from build123d import *

# Parameters (mm, degrees)
BOSS_EXTRUDE1_DEPTH = 3.175
SKETCH3_R           = 10.16
CUT_EXTRUDE1_DEPTH  = 281.570134948
LPATTERN1_COUNT     = 8
LPATTERN1_PITCH     = 35.56


with BuildPart() as part:
    # Sketch1 → Boss-Extrude1 (new body)
    with BuildSketch(Plane(origin=(0, 0, 0), x_dir=(1, 0, 0), z_dir=(0, 1, 0))):
        with BuildLine():
            Line((0, 25.4), (-254, 25.4))
            ThreePointArc((-254, 25.4), (-279.4, 0), (-254, -25.4))
            Line((-254, -25.4), (0, -25.4))
            ThreePointArc((0, -25.4), (25.4, 0), (0, 25.4))
        make_face()
    extrude(amount=BOSS_EXTRUDE1_DEPTH)

    # Sketch3 → Cut-Extrude1 (cut, through all)
    with BuildSketch(Plane(origin=(0, 3.175, 0), x_dir=(1, 0, 0), z_dir=(0, 1, 0))):
        with Locations(Location((-254, 0, 0), (0, 0, 270))):
            Circle(SKETCH3_R)
    cut_extrude1 = extrude(amount=-CUT_EXTRUDE1_DEPTH, mode=Mode.SUBTRACT)

    # LPattern1: Cut-Extrude1 ×8
    with Locations(*[(i * LPATTERN1_PITCH, 0, 0) for i in range(1, LPATTERN1_COUNT)]):
        add(cut_extrude1, mode=Mode.SUBTRACT)


solid = part.part
Verification items for the finished model (mm, model axes). Round coordinates to 2 decimals unless told otherwise and drop trailing zeros. Write each loop counter-clockwise with the first axis right and the second up, starting at its lowest first coordinate (ties: lowest second). Pieces come first, ordered by that corner, then holes.
(1) Section check D-D (x = -5.08). Enter the section's corners in (y, z) (3 decimals), plus the area to 3 significant figures.
Returned:
outline: (0, -25.4) - (3.175, -25.4) - (3.175, -10.16) - (0, -10.16) - close; (0, 10.16) - (3.175, 10.16) - (3.175, 25.4) - (0, 25.4) - close
area: 96.8 mm2
(2) Material ranges on line 1 (Z direction, x = -255, y = 1); line 2 (Z direction, x = -259, y = 1.4); line 3 (X direction, y = 1, z = -10.5), recorded low to high.
Returned:
line 1: z = -25.38 to -10.11, 10.11 to 25.38
line 2: z = -24.9 to -8.84, 8.84 to 24.9
line 3: x = -277.13 to 23.13
(3) Depth check by flat-ended pin: pin 1 Ø1.5 at (y, z) = (2.5, 1.5) entering from +X. Enter the tip coordinate at first touch or a pass-through.
Returned:
pin 1: stops at x = 25.39
(4) Section check A-A (x = -144.5). Enter the section's corners in (y, z) (3 decimals).
Returned:
outline: (0, -25.4) - (3.175, -25.4) - (3.175, -9.761) - (0, -9.761) - close; (0, 9.761) - (3.175, 9.761) - (3.175, 25.4) - (0, 25.4) - close
(5) Section check B-B (y = 1.3). Give the number of separate pieces and of enclosed holes in the cut face, plus the area to 3 significant figures.
Returned:
separate pieces: 1
enclosed holes: 8
area: 12,300 mm2
